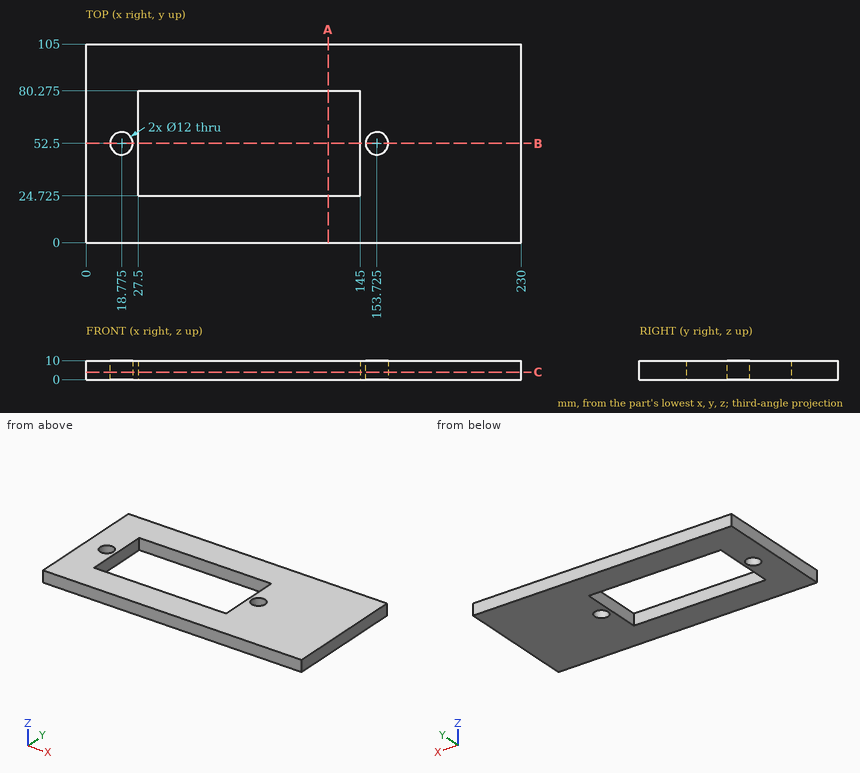
Here's the drawing with two shaded views (mm, measured from the low corner). I have some questions. Give positions to 0.01 mm unless a question says otherwise; leave off trailing zeros. Loops run counter-clockwise (first coordinate to the right, second up) from the corner with the lowest first, then second, coordinate; pieces in that order, holes last. Notation, with made-up numbers: (4, -16) - (53, -16) arc R16 ccw to (53, 6) - close; hole circle Ø10 at (44.5, -3.75). An arc over 180 degrees is marked (long way). One line per item, written item: value.
(1) I need wall thicknesses on line 1 along X through (y, z) = (29, 4.25); line 2 along Y through (x, z) = (93, 3) (3 decimals); line 3 along Y through (x, z) = (22, 2.5). Which ranges of each line are inside material? Lowest first, please.
Verdict:
line 1: 0 to 27.5, 145 to 230
line 2: 0 to 24.725, 80.275 to 105
line 3: 0 to 47.44, 57.56 to 105
(2) If we section it at C-C, the plane z = 4: List the corners of the cut face in (x, y) for me (3 decimals).
Verdict:
outline: (0, 0) - (230, 0) - (230, 105) - (0, 105) - close; hole circle Ø12 at (18.775, 52.5); hole (27.5, 24.725) - (145, 24.725) - (145, 80.275) - (27.5, 80.275) - close; hole circle Ø12 at (153.725, 52.5)
(3) If we section it at B-B, the plane y = 52.5: List the corners of the cut face in (x, z) for me (3 decimals).
Verdict:
outline: (0, 0) - (12.775, 0) - (12.775, 10) - (0, 10) - close; (24.775, 0) - (27.5, 0) - (27.5, 10) - (24.775, 10) - close; (145, 0) - (147.725, 0) - (147.725, 10) - (145, 10) - close; (159.725, 0) - (230, 0) - (230, 10) - (159.725, 10) - close
(4) If we section it at A-A, the plane x = 128: List the corners of the cut face in (y, z) for me (3 decimals), plus the area to 4 significant figures.
Verdict:
outline: (0, 0) - (24.725, 0) - (24.725, 10) - (0, 10) - close; (80.275, 0) - (105, 0) - (105, 10) - (80.275, 10) - close
area: 494.5 mm^2
